```python
from build123d import *

# Parameters (mm, degrees)
SKETCH_W     = 95
SKETCH_H     = 60
PAD_DEPTH    = 2
SKETCH001_W  = 50
SKETCH001_H  = 40
PAD001_DEPTH = 25
SKETCH002_R  = 5
PAD002_DEPTH = 53


with BuildPart() as part:
    # Sketch → Pad (new body)
    with BuildSketch(Plane.XY):
        with Locations((47.5, 30)):
            Rectangle(SKETCH_W, SKETCH_H)
    extrude(amount=PAD_DEPTH)

    # Sketch001 (on Face5 of Pad) → Pad001 (join)
    with BuildSketch(Plane(origin=(0, 0, 0), x_dir=(1, 0, 0), z_dir=(0, 0, -1))):
        with Locations((47.5, -30)):
            Rectangle(SKETCH001_W, SKETCH001_H)
    extrude(amount=PAD001_DEPTH)

    # Sketch002 (on Face5 of Pad001) → Pad002 (join)
    with BuildSketch(Plane.XY.offset(2)):
        with Locations((47.5, 30)):
            Circle(SKETCH002_R)
    extrude(amount=PAD002_DEPTH)

    # Sketch003 (on Face13 of Pad002) → Revolution (revolve)
    with BuildSketch(Plane.XY.offset(55)):
        with BuildLine():
            ThreePointArc((47.5, 50), (27.5, 30), (47.5, 10))
            Line((47.5, 50), (47.5, 10))
        make_face()
    revolve(axis=Axis((47.5, 50, 55), (0, -1, 0)))


solid = part.part
```
For this review, take the finished solid that the model builds, in its own axes (mm). A direction names the side the tool comes from. Coordinates: 2 decimals unless noted, no trailing zeros. Loops run counter-clockwise (first coordinate to the right, second up) from the corner with the lowest first, then second, coordinate; pieces in that order, holes last.
1. Add section B-B, the plane x = 47.5. Give the boundary of the cut face in (y, z), then the cut area to 3 significant figures.
2. Add section D-D, the plane y = 12. Give the boundary of the cut face in (x, z).
3. For faces 4 (the flat face through (47, 50, -12)), 5 (the flat face through (47, 10, -12)), 6 (the flat face through (72.5, 30, -12)), list the 3-axis set-ups (+Z, -Z, +X, -X, +Y, -Y) from which the entire face can be reached by the end or side of a thin tool; tool diameter is ignored.
4. Mouldability with a two-part tool opening along Z and no side actions: class faces 1 (the flat face through (22.5, 30, -12)), 2 (the flat face through (47, 30, -25)), 3 (the cylindrical face through (43.5, 27, 18.6)) as +Z half, -Z half, draft (parallel to the pull), parting line (faces both ways), or undercut.
5. Add section A-A, the plane y = 30. Give the boundary of the cut face in (x, z), then the cut area to 3 significant figures.
6. For line 1 (Z direction, x = 36, y = 31.5); line 2 (Z direction, x = 48.5, y = 52); line 3 (Z direction, x = 56, y = 29.5), list the stretches that pass through material, from the lowest coordinate up.
7. Add section C-C, the plane x = 57. Give the boundary of the cut face in (y, z), then the cut area to 3 significant figures.
8. Insertion check: P1, Ø3, axis at x = 20, y = 10, coming from the -Z side; P2, Ø4, axis at y = 36, z = 9.5, coming from the +X side; P3, Ø1.5, axis at x = 66, y = 46, coming from the +Z side; P4, Ø1.5, axis at y = 7.5, z = -1, coming from the +X side. Each pin has a flat end and moves straight along its axis. Give the tip position at first contact, or say it passes through.
Result:
1. outline: (0, 0) - (10, 0) - (10, -25) - (50, -25) - (50, 0) - (60, 0) - (60, 2) - (35, 2) - (35, 35.64) arc R20 ccw (long way) to (25, 35.64) - (25, 2) - (0, 2) - close
1. area: 2,710 mm2
2. outline: (0, 0) - (22.5, 0) - (22.5, -25) - (72.5, -25) - (72.5, 0) - (95, 0) - (95, 2) - (0, 2) - close; circle Ø17.44 at (47.5, 55)
3. face 4: -Z, +X, -X, +Y
3. face 5: -Z, +X, -X, -Y
3. face 6: -Z, +X, +Y, -Y
4. face 1: draft
4. face 2: -Z half
4. face 3: undercut
5. outline: (0, 0) - (22.5, 0) - (22.5, -25) - (72.5, -25) - (72.5, 0) - (95, 0) - (95, 2) - (52.5, 2) - (52.5, 35.64) arc R20 ccw (long way) to (42.5, 35.64) - (42.5, 2) - (0, 2) - close
5. area: 3,030 mm2
6. line 1: z = -25 to 2, 38.71 to 71.29
6. line 2: z = 0 to 2
6. line 3: z = -25 to 2, 36.9 to 73.1
7. outline: (0, 0) - (10, 0) - (10, -25) - (50, -25) - (50, 0) - (60, 0) - (60, 2) - (0, 2) - close; circle Ø35.2 at (30, 55)
7. area: 2,090 mm2
8. P1: stops at z = 0
8. P2: stops at x = 50.5
8. P3: stops at z = 2
8. P4: passes through
